Autodesk Inventor part; units mm, degrees
ref_plane "YZ Plane" through (0, 0, 0) normal (1, 0, 0) x (0, 1, 0)
ref_plane "XZ Plane" through (0, 0, 0) normal (0, 1, 0) x (-1, 0, 0)
ref_plane "XY Plane" through (0, 0, 0) normal (0, 0, 1) x (1, 0, 0)
sketch "スケッチ1" plane through (0, 0, 0) normal (0, 0, 1) x (1, 0, 0)
  line L0 (-55, -170) -> (55, -170)
  line L1 (55, -170) -> (55, 170)
  line L2 (55, 170) -> (-55, 170)
  line L3 (-55, 170) -> (-55, -170)
  line L4 (-55, -170) -> (55, 170) construction
  line L5 (55, -170) -> (-55, 170) construction
  line L6 (-55, 140) -> (-50, 140) construction
  line L7 (-50, 140) -> (-25, 165) construction
  line L8 (-25, 165) -> (-25, 170) construction
  line L9 (-46, 40.5) -> (46, 40.5) construction
  line L10 (46, 40.5) -> (46, 132.5) construction
  line L11 (46, 132.5) -> (-46, 132.5) construction
  line L12 (-46, 132.5) -> (-46, 40.5) construction
  line L13 (-46, 40.5) -> (46, 132.5) construction
  line L14 (46, 40.5) -> (-46, 132.5) construction
  line L15 (-46, 1.5) -> (46, 1.5) construction
  line L16 (46, 1.5) -> (46, 37.5) construction
  line L17 (46, 37.5) -> (-46, 37.5) construction
  line L18 (-46, 37.5) -> (-46, 1.5) construction
  line L19 (-46, 1.5) -> (46, 37.5) construction
  line L20 (46, 1.5) -> (-46, 37.5) construction
  line L21 (0, 0) -> (0, 86.5) construction
  circle A0 centre (0, 86.5) radius 53 construction
  line L22 (-44.7, 41.8) -> (44.7, 41.8) construction
  line L23 (44.7, 41.8) -> (44.7, 131.2) construction
  line L24 (44.7, 131.2) -> (-44.7, 131.2) construction
  line L25 (-44.7, 131.2) -> (-44.7, 41.8) construction
  line L26 (-44.7, 41.8) -> (44.7, 131.2) construction
  line L27 (44.7, 41.8) -> (-44.7, 131.2) construction
  arc A1 (-28.4765, 131.2) -> (-44.7, 114.9765) centre (0, 86.5) ccw
  arc A2 (-44.7, 58.0235) -> (-28.4765, 41.8) centre (0, 86.5) ccw
  arc A3 (28.4765, 41.8) -> (44.7, 58.0235) centre (0, 86.5) ccw
  arc A4 (44.7, 114.9765) -> (28.4765, 131.2) centre (0, 86.5) ccw
  line L28 (-28.4765, 131.2) -> (28.4765, 131.2)
  line L29 (-44.7, 114.9765) -> (-44.7, 58.0235)
  line L30 (-28.4765, 41.8) -> (28.4765, 41.8)
  line L31 (44.7, 58.0235) -> (44.7, 114.9765)
  line L32 (-41.25, 45.25) -> (41.25, 45.25) construction
  line L33 (41.25, 45.25) -> (41.25, 127.75) construction
  line L34 (41.25, 127.75) -> (-41.25, 127.75) construction
  line L35 (-41.25, 127.75) -> (-41.25, 45.25) construction
  line L36 (-41.25, 45.25) -> (41.25, 127.75) construction
  line L37 (41.25, 45.25) -> (-41.25, 127.75) construction
  circle A5 centre (-41.25, 127.75) radius 2.25
  circle A6 centre (-41.25, 45.25) radius 2.25
  circle A7 centre (41.25, 45.25) radius 2.25
  circle A8 centre (41.25, 127.75) radius 2.25
  circle A9 centre (-45, 160) radius 2.25
  circle A10 centre (45, 160) radius 2.25
  circle A11 centre (45, -160) radius 2.25
  circle A12 centre (-45, -160) radius 2.25
  circle A13 centre (-45, 0) radius 2.25 construction
  circle A14 centre (45, 0) radius 2.25 construction
  line L38 (-55, 0) -> (55, 0) construction
  circle A15 centre (-41.25, -49.75) radius 2.25
  arc A16 (-44.7, -36.9765) -> (-28.4765, -53.2) centre (0, -8.5) ccw
  line L39 (-28.4765, -53.2) -> (28.4765, -53.2)
  arc A17 (28.4765, -53.2) -> (44.7, -36.9765) centre (0, -8.5) ccw
  circle A18 centre (41.25, -49.75) radius 2.25
  line L40 (44.7, -36.9765) -> (44.7, 19.9765)
  circle A19 centre (41.25, 32.75) radius 2.25
  arc A20 (44.7, 19.9765) -> (28.4765, 36.2) centre (0, -8.5) ccw
  line L41 (-28.4765, 36.2) -> (28.4765, 36.2)
  circle A21 centre (-41.25, 32.75) radius 2.25
  arc A22 (-28.4765, 36.2) -> (-44.7, 19.9765) centre (0, -8.5) ccw
  line L42 (-44.7, 19.9765) -> (-44.7, -36.9765)
  circle A23 centre (-41.25, -144.75) radius 2.25
  arc A24 (-44.7, -131.9765) -> (-28.4765, -148.2) centre (0, -103.5) ccw
  line L43 (-28.4765, -148.2) -> (28.4765, -148.2)
  arc A25 (28.4765, -148.2) -> (44.7, -131.9765) centre (0, -103.5) ccw
  circle A26 centre (41.25, -144.75) radius 2.25
  line L44 (44.7, -131.9765) -> (44.7, -75.0235)
  circle A27 centre (41.25, -62.25) radius 2.25
  arc A28 (44.7, -75.0235) -> (28.4765, -58.8) centre (0, -103.5) ccw
  line L45 (-28.4765, -58.8) -> (28.4765, -58.8)
  circle A29 centre (-41.25, -62.25) radius 2.25
  arc A30 (-28.4765, -58.8) -> (-44.7, -75.0235) centre (0, -103.5) ccw
  line L46 (-44.7, -75.0235) -> (-44.7, -131.9765)
  point P0 (0, 19.5)
  point P1 (0, 19.5)
  dimension "d12" = 106
  dimension "d0" = 110
  dimension "d1" = 340
  dimension "d2" = 135
  dimension "d3" = 30
  dimension "d4" = 30
  dimension "d5" = 5
  dimension "d6" = 92
  dimension "d7" = 92
  dimension "d8" = 92
  dimension "d9" = 36
  dimension "d10" = 3
  dimension "d11" = 1.5
  dimension "d13" = 89.4
  dimension "d14" = 89.4
  dimension "d15" = 82.5
  dimension "d16" = 82.5
  dimension "d17" = 4.5
  dimension "d25" = 4.5
  dimension "d26" = 10
  dimension "d27" = 10
  dimension "d28" = 10
  dimension "d29" = 10
  dimension "d30" = 10
  dimension "d31" = 10
  dimension "d32" = 10
  dimension "d33" = 10
  dimension "d34" = 10
  dimension "d35" = 10
  dimension "d45" = 95
extrude "押し出し1" add sketch "スケッチ1" along normal blind 3 contours L3 L2 L1 L0 | A23 | L46 A30 L45 A28 L44 A25 L43 A24 | A26 | A27 | A29
sketch "スケッチ2" plane through (0, 0, 3) normal (0, 0, 1) x (1, 0, 0)
  circle A0 centre (-45, 160) radius 2.25 construction
  circle A1 centre (45, -160) radius 2.25 construction
  circle A2 centre (-45, -160) radius 2.25 construction
  circle A3 centre (-43, 158) radius 2.75 construction
  line L0 (55, 170) -> (-55, 170)
  line L1 (-55, 170) -> (-55, -170)
  line L2 (-43.7153, 161.8472) -> (-41.4298, 160.2577)
  line L3 (-45.2577, 156.4298) -> (-46.8472, 158.7153)
  circle A4 centre (-45, 160) radius 2.25 construction
  arc A5 (-43.7153, 161.8472) -> (-46.8472, 158.7153) centre (-45, 160) ccw
  arc A6 (-45.2577, 156.4298) -> (-41.4298, 160.2577) centre (-43, 158) ccw
  line L4 (55, 170) -> (-55, 170) construction
  line L5 (0, 170) -> (0, -170) construction
  line L6 (-55, -170) -> (55, -170) construction
  line L7 (-55, 0) -> (55, 0) construction
  line L8 (55, -170) -> (55, 170) construction
  circle A7 centre (45, 160) radius 2.25 construction
  circle A8 centre (43, 158) radius 2.75 construction
  line L9 (43.7153, 161.8472) -> (41.4298, 160.2577)
  line L10 (45.2577, 156.4298) -> (46.8472, 158.7153)
  circle A9 centre (45, 160) radius 2.25 construction
  arc A10 (46.8472, 158.7153) -> (43.7153, 161.8472) centre (45, 160) ccw
  arc A11 (41.4298, 160.2577) -> (45.2577, 156.4298) centre (43, 158) ccw
  circle A12 centre (-45, -160) radius 2.25 construction
  circle A13 centre (-43, -158) radius 2.75 construction
  line L11 (-43.7153, -161.8472) -> (-41.4298, -160.2577)
  line L12 (-45.2577, -156.4298) -> (-46.8472, -158.7153)
  circle A14 centre (-45, -160) radius 2.25 construction
  arc A15 (-46.8472, -158.7153) -> (-43.7153, -161.8472) centre (-45, -160) ccw
  arc A16 (-41.4298, -160.2577) -> (-45.2577, -156.4298) centre (-43, -158) ccw
  circle A17 centre (45, -160) radius 2.25 construction
  line L13 (45.2577, -156.4298) -> (46.8472, -158.7153)
  arc A18 (45.2577, -156.4298) -> (41.4298, -160.2577) centre (43, -158) ccw
  circle A19 centre (43, -158) radius 2.75 construction
  line L14 (43.7153, -161.8472) -> (41.4298, -160.2577)
  circle A20 centre (45, -160) radius 2.25 construction
  arc A21 (43.7153, -161.8472) -> (46.8472, -158.7153) centre (45, -160) ccw
  point P0 (0, 0)
  dimension "d38" = 5.5
  dimension "d39" = 12
  dimension "d40" = 12
extrude "押し出し2" cut sketch "スケッチ2" against normal through all
sketch "スケッチ3" plane through (0, 0, 3) normal (0, 0, 1) x (1, 0, 0)
  line L0 (-55, -170) -> (55, -170) construction
  line L1 (-55, 170) -> (-55, -170) construction
  line L2 (55, -170) -> (55, 170) construction
  line L3 (0, -170) -> (0, -116.79) construction
  arc A0 (-17.4739, -147.55) -> (-17.4739, -162.45) centre (-15, -155) ccw construction
  line L4 (-17.4739, -147.55) -> (-12.5261, -147.55) construction
  line L5 (-12.5261, -162.45) -> (-17.4739, -162.45) construction
  arc A1 (-12.5261, -147.55) -> (-17.4739, -147.55) centre (-15, -155) ccw construction
  arc A2 (-12.5261, -162.45) -> (-12.5261, -147.55) centre (-15, -155) ccw construction
  arc A3 (-17.4739, -162.45) -> (-12.5261, -162.45) centre (-15, -155) ccw construction
  line L6 (-17.4755, -162.46) -> (-12.5245, -162.46)
  arc A4 (-12.5245, -162.46) -> (-12.5245, -147.54) centre (-15, -155) ccw
  line L7 (-12.5245, -147.54) -> (-17.4755, -147.54)
  arc A5 (-17.4755, -147.54) -> (-17.4755, -162.46) centre (-15, -155) ccw
  line L8 (17.4755, -162.46) -> (12.5245, -162.46)
  arc A6 (12.5245, -147.54) -> (12.5245, -162.46) centre (15, -155) ccw
  line L9 (12.5245, -147.54) -> (17.4755, -147.54)
  arc A7 (17.4755, -162.46) -> (17.4755, -147.54) centre (15, -155) ccw
  point P0 (0, 0)
  dimension "d50" = 15.7
  dimension "d51" = 14.9
  dimension "d52" = 15
  dimension "d53" = 15
  dimension "d54" = 40
  dimension "d55" = 0.01
extrude "押し出し3" cut sketch "スケッチ3" against normal through all
sketch "スケッチ4" plane through (0, 0, 3) normal (0, 0, 1) x (1, 0, 0)
  line L0 (-55, 170) -> (-55, -170)
  line L1 (-55, 170) -> (55, 170)
  line L2 (55, 170) -> (55, 167)
  line L3 (55, 167) -> (-55, 167)
  line L4 (-55, 167) -> (-55, 170)
  point P0 (0, 0)
  dimension "d58" = 3
extrude "押し出し4" [suppressed]
equation "\"d4\" = d3"
equation "\"d11\" = 0.5 * d10"
equation "\"d27\" = d26"
equation "\"d28\" = d26"
equation "\"d29\" = d26"
equation "\"d30\" = d26"
equation "\"d31\" = d26"
equation "\"d32\" = d26"
equation "\"d33\" = d26"
equation "\"d34\" = d26"
equation "\"d35\" = d26"
equation "\"d45\" = d7 + d10"
properties part number "top_panel" material "アルミニウム 6061"
Input: part model. Units: mm. Frame: model coordinates. A direction names the side the tool comes from. Coordinates: 2 decimals unless noted, no trailing zeros. Order: outer loops, then holes, each group sorted by start corner. A loop starts at its lowest first (then second) coordinate and runs counter-clockwise, first axis right, second up. Notation, with made-up numbers: M 41,87 L 53,87 A24 cw 53,111 Z; hole C -7,47.25 d4. An arc over 180 degrees is marked long. Answer in a Markdown table with one row per item.
(1) Contact query for a flat-ended pin moving along its axis: pin 1 Ø6 at (x, y) = (-41.25, 45.25) entering from -Z. Output: stop coordinate, or through.
Numbers:
| item | result |
|---|---|
| pin 1 | stops at z = 0 |
(2) Section query A-A, the plane y = 99. Output: boundary loops of the cut face in (x, z), plus the area to 3 significant figures.
Numbers:
| item | result |
|---|---|
| outline | M -55,0 L -44.7,0 L -44.7,3 L -55,3 Z; M 44.7,0 L 55,0 L 55,3 L 44.7,3 Z |
| area | 61.8 mm^2 |
(3) Draft query along X for faces 3 (the flat face through (-50, 2, 3)), 4 (the cylindrical face through (-7.14, -155.14, 1.52)). Return one class per face: pulls with the +X half, pulls with the -X half, needs draft (parallel to the pull), parting line crosses it, or undercut.
Numbers:
| item | result |
|---|---|
| face 3 | needs draft |
| face 4 | undercut |
(4) Material intervals for line 1 (Y direction, x = -14, z = 1.25); line 2 (Y direction, x = 36, z = 2.25); line 3 (Y direction, x = -7, z = 2.45), sorted ascending. Write a range as [from, to].
Numbers:
| item | result |
|---|---|
| line 1 | y = [-170, -162.46], [-147.54, -53.2], [36.2, 41.8], [131.2, 170] |
| line 2 | y = [-170, -47.4], [30.4, 47.6], [125.4, 170] |
| line 3 | y = [-170, -53.2], [36.2, 41.8], [131.2, 170] |
(5) Access query for faces 1 (the flat face through (-50, 2, 0)), 2 (the cylindrical face through (-37.591, 123.862, 1.479)). Directions: +Z, -Z, +X, -X, +Y, -Y. A direction counts if a zero-diameter tool reaches every point of the face in a straight line with its end or side. Return the directions, or none.
Numbers:
| item | result |
|---|---|
| face 1 | -Z, +X, -X, +Y, -Y |
| face 2 | +Z, -Z |
(6) Section query B-B, the plane z = 1.55. Give the number of separate pieces and of enclosed holes in the cut face, plus the area to 3 significant figures.
Numbers:
| item | result |
|---|---|
| separate pieces | 1 |
| enclosed holes | 16 |
| area | 21,700 mm^2 |
